Here's how the part is built. I have some questions about the finished solid (model axes, mm). Face numbers are marked on the shaded views. A direction names the side the tool comes from. Give positions to 0.01 mm unless a question says otherwise; leave off trailing zeros. Order: outer loops, then holes, each group sorted by start corner. A loop starts at its lowest first (then second) coordinate and runs counter-clockwise, first axis right, second up. Notation, with made-up numbers: M -23,64.5 L 32,64.5 A27 cw 32,83.5 Z; hole C 35.5,89 d6. An arc over 180 degrees is marked long. One line per item, written item: value. Start each with the question number.
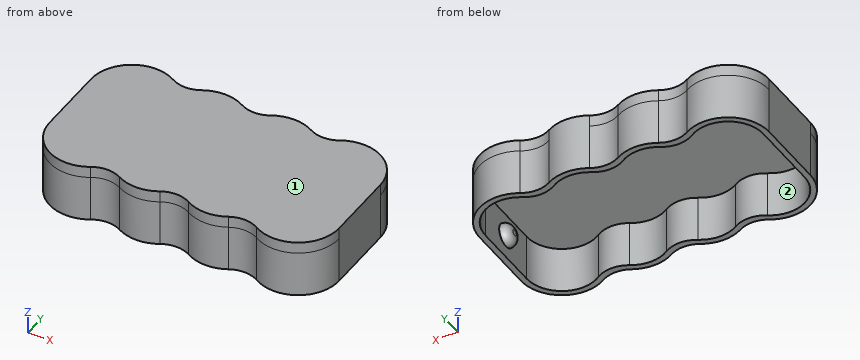
from build123d import *

# Parameters (mm, degrees)
F1_DEPTH  = 8
F2_R      = 5
F3_R      = 5.1
F5_DEPTH  = 2
F6_R      = 2
F7_DEPTH  = 1.5
F8_R      = 1.49999
F9_R      = 2
F10_DEPTH = 1.5
F11_R     = 1.49999


# Not quite as in the source:
# - a fillet or chamfer is up to 0.001 mm smaller than in the source, because OpenCascade refuses the exact size


with BuildPart() as f1:
    # F0 (on Top) → F1 (new body)
    with BuildSketch(Plane.XY):
        with BuildLine():
            ThreePointArc((0, 9.7960505792), (-5.9794748492, 13.0999703322), (-11.9779520569, 9.830677382))
            ThreePointArc((-11.9779520569, 9.830677382), (-19.9562029041, 12.8948954194), (-25.1, 6.0697016347))
            Line((-25.1, 6.0697016347), (-25.1, -6.0697016347))
            ThreePointArc((-25.1, -6.0697016347), (-19.9296547743, -12.9024486996), (-11.9488922671, -9.7837419151))
            ThreePointArc((-11.9488922671, -9.7837419151), (-5.9300692346, -12.9669396851), (0, -9.6213070677))
            ThreePointArc((0, -9.6213070677), (5.9300692346, -12.9669396851), (11.9488922671, -9.7837419151))
            ThreePointArc((11.9488922671, -9.7837419151), (19.9296547743, -12.9024486996), (25.1, -6.0697016347))
            Line((25.1, -6.0697016347), (25.1, 6.0697016347))
            ThreePointArc((25.1, 6.0697016347), (19.9562029041, 12.8948954194), (11.9779520569, 9.830677382))
            ThreePointArc((11.9779520569, 9.830677382), (5.9794748492, 13.0999703322), (0, 9.7960505792))
        make_face()
        with BuildLine():
            ThreePointArc((-24.1, 6.0697016347), (-18.5343432382, 12.1462530666), (-11.9936139988, 7.1342800509))
            ThreePointArc((-11.9936139988, 7.1342800509), (-5.9825651004, 12.0999750839), (0, 7.1))
            ThreePointArc((0, 7.1), (5.9825651004, 12.0999750839), (11.9936139988, 7.1342800509))
            ThreePointArc((11.9936139988, 7.1342800509), (18.5343432382, 12.1462530666), (24.1, 6.0697016347))
            Line((24.1, 6.0697016347), (24.1, -6.0697016347))
            ThreePointArc((24.1, -6.0697016347), (18.5343432382, -12.1462530666), (11.9936139988, -7.1342800509))
            ThreePointArc((11.9936139988, -7.1342800509), (5.8623077698, -11.9653833554), (0, -6.8111789722))
            ThreePointArc((0, -6.8111789722), (-5.8623077698, -11.9653833554), (-11.9936139988, -7.1342800509))
            ThreePointArc((-11.9936139988, -7.1342800509), (-18.5343432382, -12.1462530666), (-24.1, -6.0697016347))
            Line((-24.1, -6.0697016347), (-24.1, 6.0697016347))
        make_face(mode=Mode.SUBTRACT)
    extrude(amount=F1_DEPTH)

    # F2
    f2_edges = [f1.edges().sort_by_distance(p)[0] for p in [
        (-11.948892, -9.783742, 4),
        (0, -9.621307, 4),
        (11.948892, -9.783742, 4),
        (-11.977952, 9.830677, 4),
        (0, 9.796051, 4),
        (11.977952, 9.830677, 4),
    ]]
    fillet(f2_edges, radius=F2_R)

    # F3
    f3_edges = [f1.edges().sort_by_distance(p)[0] for p in [
        (-11.993614, -7.13428, 4),
        (0, -6.811179, 4),
        (11.993614, -7.13428, 4),
        (11.993614, 7.13428, 4),
        (0, 7.1, 4),
        (-11.993614, 7.13428, 4),
    ]]
    fillet(f3_edges, radius=F3_R)

    # F4 (on face) → F5 (join)
    with BuildSketch(Plane.XY.offset(8)):
        with BuildLine():
            ThreePointArc((-9.4848491067, 12.1859378193), (-11.9680100538, 11.5423164018), (-14.4435267926, 12.2147401477))
            ThreePointArc((-14.4435267926, 12.2147401477), (-21.5467619195, 12.2203503717), (-25.1, 6.0697016347))
            Line((-25.1, 6.0697016347), (-25.1, -6.0697016347))
            ThreePointArc((-25.1, -6.0697016347), (-21.5163446166, -12.2377905233), (-14.3830082993, -12.179314637))
            ThreePointArc((-14.3830082993, -12.179314637), (-11.9202167891, -11.4825711508), (-9.4353135356, -12.0957997614))
            ThreePointArc((-9.4353135356, -12.0957997614), (-5.9534768613, -12.9672192968), (-2.4903217652, -12.0242901298))
            ThreePointArc((-2.4903217652, -12.0242901298), (0, -11.3599904776), (2.4903217652, -12.0242901298))
            ThreePointArc((2.4903217652, -12.0242901298), (5.9534768613, -12.9672192968), (9.4353135356, -12.0957997614))
            ThreePointArc((9.4353135356, -12.0957997614), (11.9202167891, -11.4825711508), (14.3830082993, -12.179314637))
            ThreePointArc((14.3830082993, -12.179314637), (21.5163446166, -12.2377905233), (25.1, -6.0697016347))
            Line((25.1, -6.0697016347), (25.1, 6.0697016347))
            ThreePointArc((25.1, 6.0697016347), (21.5467619195, 12.2203503717), (14.4435267926, 12.2147401477))
            ThreePointArc((14.4435267926, 12.2147401477), (11.9680100538, 11.5423164018), (9.4848491067, 12.1859378193))
            ThreePointArc((9.4848491067, 12.1859378193), (5.9794143891, 13.0999701572), (2.479338843, 12.1656260848))
            ThreePointArc((2.479338843, 12.1656260848), (0, 11.5076162853), (-2.479338843, 12.1656260848))
            ThreePointArc((-2.479338843, 12.1656260848), (-5.9794143891, 13.0999701572), (-9.4848491067, 12.1859378193))
        make_face()
    extrude(amount=F5_DEPTH)

    # F6 (on face) → F7 (join)
    with BuildSketch(Plane.YZ.offset(-24.1)):
        with Locations((0, 4)):
            Circle(F6_R)
    extrude(amount=F7_DEPTH)

    # F8 (radius 1.5 in the source; OpenCascade refuses exactly that, so slightly less here)
    f8_edges = [f1.edges().sort_by_distance(p)[0] for p in [
        (-22.6, -2, 4),
    ]]
    fillet(f8_edges, radius=F8_R)

    # F9 (on face) → F10 (join)
    with BuildSketch(Plane(origin=(24.1, 0, 0), x_dir=(0, -1, 0), z_dir=(-1, 0, 0))):
        with Locations((0, 4)):
            Circle(F9_R)
    extrude(amount=F10_DEPTH)

    # F11 (radius 1.5 in the source; OpenCascade refuses exactly that, so slightly less here)
    f11_edges = [f1.edges().sort_by_distance(p)[0] for p in [
        (22.6, 2, 4),
    ]]
    fillet(f11_edges, radius=F11_R)


solid = f1.part
Item 1: For the marked faces 1 and 2, which set-ups out of +Z, -Z, +X, -X, +Y, -Y let a thin tool reach every point of the face, with its end or its side?
Item 2: I want a section at D-D on x = -16.5. Write out the boundary of the cut face in (y, z), plus the area to 3 significant figures.
Item 3: Please list where these lines run through material, in increasing order: probe 1 along X at (y, z) = (4.25, 1.5); probe 2 along Y at (x, z) = (-18, 5); probe 3 along Y at (x, z) = (6, 3.75). Write a range as [from, to].
Item 4: Will these pins go through, and if not, where does the flat tip stop? P1, Ø10, axis at x = 1, y = -0.5, coming from the -Z side; P2, Ø1, axis at x = -7, z = 3.5, coming from the -Y side.
Item 5: I want a section at A-A on y = 3. Write out the boundary of the cut face in (x, z), plus the area to 3 significant figures.
Item 6: I want a section at B-B on z = 9.25. Write out the boundary of the cut face in (x, y), plus the area to 3 significant figures.
Item 7: I want a section at C-C on x = 8.5. Write out the boundary of the cut face in (y, z).
Answer below:
1. face 1: +Z, +X, -X, +Y, -Y
1. face 2: -Z
2. outline: M -13.01,0 L -11.98,0 L -11.98,8 L 11.98,8 L 11.98,0 L 13.01,0 L 13.01,10 L -13.01,10 Z
2. area: 68.5 mm²
3. probe 1: x = [-25.1, -24.1], [24.1, 25.1]
3. probe 2: y = [-13.17, -12.17], [12.17, 13.17]
3. probe 3: y = [-12.97, -11.97], [12.1, 13.1]
4. P1: stops at z = 8
4. P2: stops at y = -12.95
5. outline: M -25.1,0 L -24.1,0 L -24.1,8 L 24.1,8 L 24.1,0 L 25.1,0 L 25.1,10 L -25.1,10 Z
5. area: 116 mm²
6. outline: M -25.1,-6.07 A7.1 ccw -14.38,-12.18 A5 cw -9.44,-12.1 A7.1 ccw -2.49,-12.02 A5 cw 2.49,-12.02 A7.1 ccw 9.44,-12.1 A5 cw 14.38,-12.18 A7.1 ccw 25.1,-6.07 L 25.1,6.07 A7.1 ccw 14.44,12.21 A5 cw 9.48,12.19 A7.1 ccw 2.48,12.17 A5 cw -2.48,12.17 A7.1 ccw -9.48,12.19 A5 cw -14.44,12.21 A7.1 ccw -25.1,6.07 Z
6. area: 1,220 mm²
7. outline: M -12.52,0 L -11.44,0 L -11.44,8 L 11.56,8 L 11.56,0 L 12.65,0 L 12.65,10 L -12.52,10 Z
